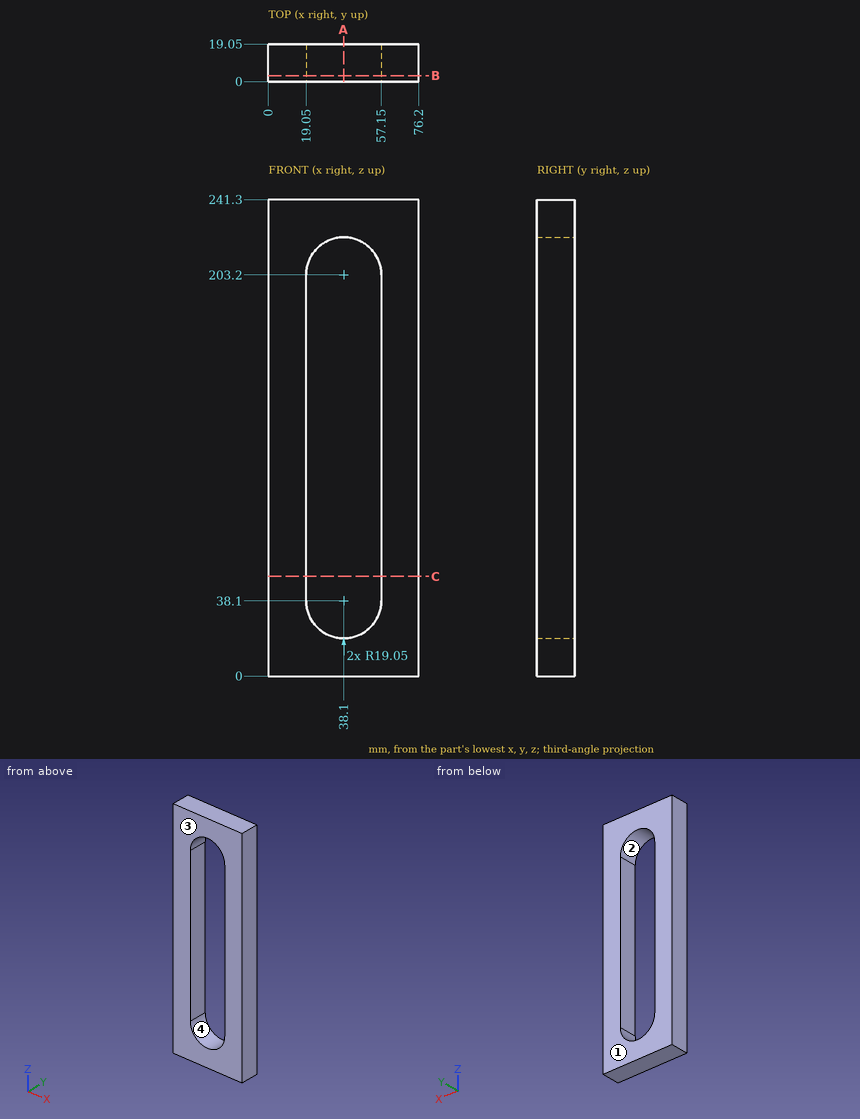
The drawing under review shows one solid part. Ordinate dimensions are in mm from its lowest x, y, z. A direction names the side the tool comes from. Coordinates: 2 decimals unless noted, no trailing zeros. Write each loop counter-clockwise with the first axis right and the second up, starting at its lowest first coordinate (ties: lowest second). Pieces come first, ordered by that corner, then holes. Notation, with made-up numbers: (12, 0.25) -> (43, 0.25) arc R17 ccw to (43, 19.25) -> close; hole circle Ø9 at (62.25, 45). An arc over 180 degrees is marked (long way). Write each question's results on one line, items separated by ' | '. Start each with the question number.
1) The part is to be moulded in two halves that separate along Z. For the marked faces 3 and 4, say which applies: +Z half, -Z half, draft (parallel to the pull), parting line (faces both ways), or undercut.
2) Wall thickness on L1, parallel to X at y = 1.5, z = 121; L2, parallel to X at y = 18.25, z = 204.5; L3, parallel to Z at x = 38, y = 13.5: over which ranges is each line inside the solid? List them lowest first. Write a range as [from, to].
3) Consider section C-C (z = 50.5). Write out the cut boundary in (x, y).
4) Consider section A-A (x = 38.1). Write out the cut boundary in (y, z).
5) Consider section B-B (y = 3). Write out the cut boundary in (x, z), plus the area to 3 significant figures.
6) For the marked faces 1 and 2, list the 3-axis set-ups (+Z, -Z, +X, -X, +Y, -Y) from which the entire face can be reached by the end or side of a thin tool; tool diameter is ignored.
Geometry says:
1) face 3: draft | face 4: undercut
2) L1: [0, 19.05], [57.15, 76.2] | L2: [0, 19.09], [57.11, 76.2] | L3: [0, 19.05], [222.25, 241.3]
3) outline: (0, 0) -> (19.05, 0) -> (19.05, 19.05) -> (0, 19.05) -> close; (57.15, 0) -> (76.2, 0) -> (76.2, 19.05) -> (57.15, 19.05) -> close
4) outline: (0, 0) -> (19.05, 0) -> (19.05, 19.05) -> (0, 19.05) -> close; (0, 222.25) -> (19.05, 222.25) -> (19.05, 241.3) -> (0, 241.3) -> close
5) outline: (0, 0) -> (76.2, 0) -> (76.2, 241.3) -> (0, 241.3) -> close; hole (19.05, 38.1) arc R19.05 ccw to (57.15, 38.1) -> (57.15, 203.2) arc R19.05 ccw to (19.05, 203.2) -> close | area: 11,000 mm^2
6) face 1: +Z, -Z, +X, -X, +Y | face 2: +Y, -Y
